```python
from build123d import *

# Parameters (mm, degrees)
F2_R            = 63.5
F2_R_2          = 6.35
F3_DEPTH        = 53.849
F3_COPIES_COUNT = 4
F4_R            = 2


# Not quite as in the source:
# - a pattern or mirror of a feature is missing from the dataset's text; its kind, count and spacing are read off the source's solid
# - a feature names something its author has since deleted; it is built from what else it names


with BuildPart() as f1:
    # F0 (on Right) → F1 (revolve)
    with BuildSketch(Plane.YZ):
        Polygon((-53.848, 19.05), (0, 19.05), (0, 69.85), (-19.05, 69.85), (-19.05, 35.052), (-53.848, 35.052), align=None)
    revolve(axis=Axis((0, -26.924, 0), (0, -1, 0)))

    # F2 (on Front) → F3 (cut, through all)
    with BuildSketch(Plane.XZ):
        with Locations((0, 265.2071825894)):
            Circle(F2_R)
        with Locations((0, 53.848)):
            Circle(F2_R_2)
    f3 = extrude(amount=F3_DEPTH, mode=Mode.SUBTRACT)

    # F3_copies: F3 ×4 about axis
    f3_copies_axis = Axis((0, 0, 0), (0, 1, 0))
    for i in range(1, F3_COPIES_COUNT):
        add(f3.rotate(f3_copies_axis, i * 360 / F3_COPIES_COUNT), mode=Mode.SUBTRACT)

    # F4
    f4_edges = [f1.edges().sort_by_distance(p)[0] for p in [
        (0, -19.05, -69.85),
        (0, -19.05, -35.052),
        (0, -53.848, -35.052),
    ]]
    fillet(f4_edges, radius=F4_R)


solid = f1.part
```
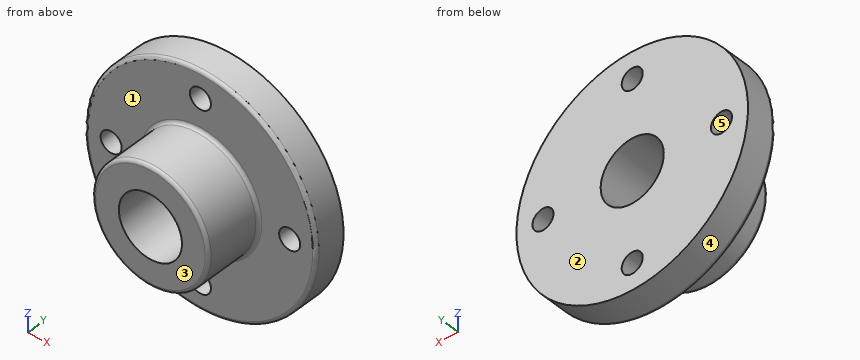
The listing builds one solid part. Answer for the finished solid, in the listing's coordinates (mm). Face numbers are marked on the shaded views. A direction names the side the tool comes from. Coordinates: 2 decimals unless noted, no trailing zeros. Write each loop counter-clockwise with the first axis right and the second up, starting at its lowest first coordinate (ties: lowest second). Pieces come first, ordered by that corner, then holes. Notation, with made-up numbers: (89.25, -10) - (123.25, -10) arc R12 ccw to (123.25, 1) - close; hole circle Ø7 at (-5.75, 67.25). An arc over 180 degrees is marked (long way). Return JSON: item names as keys, results as strings. Group by question number.
1. Straight lines are drawn through the part: L1, parallel to Z at x = 0, y = -4; L2, parallel to Z at x = 1, y = -24.5. For each, find the intervals that lie inside material, in ascending order.
2. A cutting plane is placed at A-A, the plane x = 0. Determine the outline of the cut face in (y, z).
3. A cutting plane is placed at C-C, the plane y = -43. Determine the outline of the cut face in (x, z).
4. Given pin 1 (16.5 mm diameter, centred on x = -53.848, z = 0, fed in from -Y); pin 2 (10 mm diameter, centred on y = -23.5, z = -0.5, fed in from +X); pin 3 (4 mm diameter, centred on x = 11.5, y = -46, fed in from +Z); pin 4 (16.5 mm diameter, centred on x = 0, z = 53.848, fed in from +Y), each flat-ended and moving along its own axis, determine where each tip first touches the part or whether it passes through.
5. Determine the mould class of the marked faces 3, 4 and 5 for opening direction Z: released by +Z, released by -Z, zero draft, split by the parting line, or undercut.
6. Which of the six approach directions +Z, -Z, +X, -X, +Y, -Y give full straight-line access (tool end or side, diameter ignored) to the marked faces 1 and 2?
7. A cutting plane is placed at B-B, the plane z = 0. Determine the outline of the cut face in (x, y).
Ans:
{
 "1": {"L1": "-69.85 to -60.2, -47.5 to -19.05, 19.05 to 47.5, 60.2 to 69.85", "L2": "-35.04 to -19.02, 19.02 to 35.04"},
 "2": {"outline": "(-53.85, -33.05) arc R2 ccw to (-51.85, -35.05) - (-21.05, -35.05) arc R2 cw to (-19.05, -37.05) - (-19.05, -47.5) - (0, -47.5) - (0, -19.05) - (-53.85, -19.05) - close; (-53.85, 19.05) - (0, 19.05) - (0, 47.5) - (-19.05, 47.5) - (-19.05, 37.05) arc R2 cw to (-21.05, 35.05) - (-51.85, 35.05) arc R2 ccw to (-53.85, 33.05) - close; (-19.05, -67.85) arc R2 ccw to (-17.05, -69.85) - (0, -69.85) - (0, -60.2) - (-19.05, -60.2) - close; (-19.05, 60.2) - (0, 60.2) - (0, 69.85) - (-17.05, 69.85) arc R2 ccw to (-19.05, 67.85) - close"},
 "3": {"outline": "circle Ø70.1 at (0, 0); hole circle Ø38.1 at (0, 0)"},
 "4": {"pin 1": "y = -19.05", "pin 2": "x = 69.23", "pin 3": "z = 33.74", "pin 4": "y = 0"},
 "5": {"face 3": "zero draft", "face 4": "split by the parting line", "face 5": "undercut"},
 "6": {"face 1": "-Y", "face 2": "+Z, -Z, +X, -X, +Y"},
 "7": {"outline": "(-69.85, -17.05) arc R2 ccw to (-67.85, -19.05) - (-60.2, -19.05) - (-60.2, 0) - (-69.85, 0) - close; (-47.5, -19.05) - (-37.05, -19.05) arc R2 cw to (-35.05, -21.05) - (-35.05, -51.85) arc R2 ccw to (-33.05, -53.85) - (-19.05, -53.85) - (-19.05, 0) - (-47.5, 0) - close; (19.05, -53.85) - (33.05, -53.85) arc R2 ccw to (35.05, -51.85) - (35.05, -21.05) arc R2 cw to (37.05, -19.05) - (47.5, -19.05) - (47.5, 0) - (19.05, 0) - close; (60.2, -19.05) - (67.85, -19.05) arc R2 ccw to (69.85, -17.05) - (69.85, 0) - (60.2, 0) - close"}
}
